Here's how the part is built. I have some questions about the finished solid (model axes, mm). Face numbers are marked on the shaded views. A direction names the side the tool comes from. Give positions to 0.01 mm unless a question says otherwise; leave off trailing zeros. Loops run counter-clockwise (first coordinate to the right, second up) from the corner with the lowest first, then second, coordinate; pieces in that order, holes last.
Q1. For the marked faces 1 and 2, which set-ups out of +Z, -Z, +X, -X, +Y, -Y let a thin tool reach every point of the face, with its end or its side?
Q2. I need wall thicknesses on probe 1 along Z at (x, y) = (-23.25, 4.5); probe 2 along Y at (x, z) = (-18, 0.2); probe 3 along X at (y, z) = (7.5, -0.3). Which ranges of each line are inside material? Lowest first, please.
Q3. Suppose I cut it at A-A (z = -0.6). Count the separate pieces of the cut face and the enclosed holes in it, and give its area (3 significant figures).
Q4. I'm going to push flat-ended pins straight in: P1, Ø3.5, axis at x = -12, y = 6, coming from the -Z side; P2, Ø1, axis at y = 2, z = -0.5, coming from the -X side; P3, Ø1.5, axis at x = -17, y = -8, coming from the +Z side. Where does each tip first touch, or does it pass through?
Q5. Suppose I cut it at C-C (x = -13.75). List the corners of the cut face in (y, z) for me, and give its area (3 significant figures).
Q6. Suppose I cut it at D-D (z = 1.15). List the corners of the cut face in (x, y) for me, and give its area (3 significant figures).
Q7. Suppose I cut it at B-B (y = 9). List the corners of the cut face in (x, z) for me.
```python
from build123d import *

# Parameters (mm, degrees)
SALIENTE_EXTRUIR2_START       = -1.018233765
SALIENTE_EXTRUIR2_OUTLINE_R   = 0.509116882
SALIENTE_EXTRUIR2_OUTLINE_R_2 = 0.763675324
SALIENTE_EXTRUIR2_DEPTH       = 1.018233765
CROQUIS2_R                    = 0.509116882
SALIENTE_EXTRUIR3_DEPTH       = 1.8


# Read off the part's stored shape, not the designer's step: Saliente-Extruir2
with BuildPart() as part:
    # Saliente-Extruir2 outline → Saliente-Extruir2 (new body)
    # profile 1 of 2: a face of its own
    with BuildSketch(Plane.XY.offset(SALIENTE_EXTRUIR2_START)):
        with BuildLine():
            ThreePointArc((-7.817662351, 0), (-15.017662351, 2.982337649), (-18, 10.182337649))
            ThreePointArc((-18, 10.182337649), (-25.2, -7.2), (-7.817662351, 0))
        make_face()
        with Locations((-18, 0)):
            Circle(SALIENTE_EXTRUIR2_OUTLINE_R, mode=Mode.SUBTRACT)
    # profile 2 of 2: a face of its own
    with BuildSketch(Plane.XY.offset(SALIENTE_EXTRUIR2_START)):
        with Locations((-9, 9)):
            Circle(SALIENTE_EXTRUIR2_OUTLINE_R_2)
        with BuildLine():
            Line((-8.64, 9.36), (-8.632797118, 9.352797118))
            ThreePointArc((-8.632797118, 9.352797118), (-8.64, 8.64), (-9.352727993, 8.632872007))
            Line((-9.352727993, 8.632872007), (-9.36, 8.64))
            ThreePointArc((-9.36, 8.64), (-9.36, 9.36), (-8.64, 9.36))
        make_face(mode=Mode.SUBTRACT)
    extrude(amount=SALIENTE_EXTRUIR2_DEPTH)

    # Croquis2 → Saliente-Extruir3 (add)
    with BuildSketch(Plane.XY):
        with BuildLine():
            Line((-17.265744014, -0.705455986), (-8.449308011, 8.470908011))
            ThreePointArc((-8.449308011, 8.470908011), (-8.46, 9.54), (-9.529091989, 9.550691989))
            Line((-9.529091989, 9.550691989), (-18.705455986, 0.734255986))
            ThreePointArc((-18.705455986, 0.734255986), (-18.72, -0.72), (-17.265744014, -0.705455986))
        make_face()
        with Locations((-18, 0)):
            Circle(CROQUIS2_R, mode=Mode.SUBTRACT)
    extrude(amount=SALIENTE_EXTRUIR3_DEPTH)


solid = part.part
```
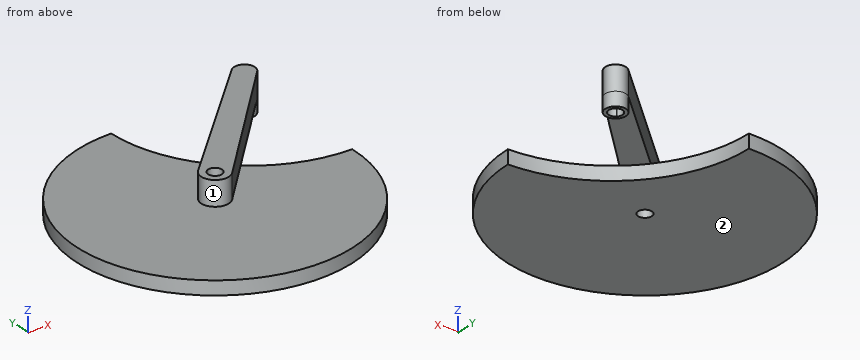
Solutions:
1. face 1: +Z
1. face 2: -Z, +X, -X, +Y, -Y
2. probe 1: z = -1.02 to 0
2. probe 2: y = -1.02 to -0.51, 0.51 to 1.41
2. probe 3: x = -24.89 to -17.64
3. separate pieces: 2
3. enclosed holes: 2
3. area: 267 mm2
4. P1: stops at z = 0
4. P2: stops at x = -28.07
4. P3: stops at z = 0
5. outline: (-9.25, -1.02) - (1.91, -1.02) - (1.91, 0) - (-9.25, 0) - close; (2.95, 0) - (5.5, 0) - (5.5, 1.8) - (2.95, 1.8) - close
5. area: 15.9 mm2
6. outline: (-18.71, 0.73) arc R1.02 ccw (long way) to (-17.27, -0.71) - (-8.45, 8.47) arc R0.76 ccw to (-9.53, 9.55) - close; hole circle Ø1.02 at (-18, 0)
6. area: 24.4 mm2
7. outline: (-22.76, -1.02) - (-17.93, -1.02) - (-17.93, 0) - (-22.76, 0) - close; (-10.1, 0) - (-9.76, 0) - (-9.76, -1.02) - (-9.51, -1.02) - (-9.51, 0) - (-8.49, 0) - (-8.49, -1.02) - (-8.24, -1.02) - (-8.24, 1.8) - (-10.1, 1.8) - close
